from build123d import *

# Parameters (mm, degrees)
CIRCLE001_R            = 0.99
EXTRUDE060_DEPTH       = 4
CIRCLE002_R            = 0.98
EXTRUDE059_DEPTH       = 4
CIRCLE003_R            = 0.99
EXTRUDE058_DEPTH       = 4
CIRCLE004_R            = 0.98
EXTRUDE057_DEPTH       = 4
CIRCLE051_R            = 3.5
EXTRUDE056_DEPTH       = 1.5
EXTRUDE055_DEPTH       = 2.5
CIRCLE049_R            = 2.6
EXTRUDE052_DEPTH       = 1.5
CIRCLE048_R            = 2.6
EXTRUDE051_DEPTH       = 1.5
CIRCLE047_R            = 2.6
EXTRUDE050_DEPTH       = 1.5
CIRCLE050_R            = 2.6
EXTRUDE049_DEPTH       = 1.5
CIRCLE045_R            = 1.5
EXTRUDE045_DEPTH       = 4
CIRCLE043_R            = 1.5
EXTRUDE046_DEPTH       = 4
CIRCLE046_R            = 1.5
EXTRUDE047_DEPTH       = 4
CIRCLE044_R            = 1.5
EXTRUDE048_DEPTH       = 4
CIRCLE040_R            = 23.5
EXTRUDE044_DEPTH       = 4
CUT015_PLACEMENT_ANGLE = 45
CUT018_PLACEMENT_ANGLE = 180


with BuildPart() as extrude060:
    # Circle001 → Extrude060 (new body)
    with BuildSketch(Plane(origin=(100.138196, 1.761986, -7), x_dir=(1, 0, 0), z_dir=(0, 0, -1))):
        Circle(CIRCLE001_R)
    extrude(amount=-EXTRUDE060_DEPTH)


with BuildPart() as extrude059:
    # Circle002 (on Circle) → Extrude059 (new body)
    with BuildSketch(Plane(origin=(104.140973, 1.752854, -7), x_dir=(1, 0, 0), z_dir=(0, 0, -1))):
        Circle(CIRCLE002_R)
    extrude(amount=-EXTRUDE059_DEPTH)


with BuildPart() as extrude058:
    # Circle003 (on Circle) → Extrude058 (new body)
    with BuildSketch(Plane(origin=(121.638501, 1.757256, -7), x_dir=(1, 0, 0), z_dir=(0, 0, -1))):
        Circle(CIRCLE003_R)
    extrude(amount=-EXTRUDE058_DEPTH)


with BuildPart() as extrude057:
    # Circle004 → Extrude057 (new body)
    with BuildSketch(Plane(origin=(125.641919, 1.759529, -7), x_dir=(1, 0, 0), z_dir=(0, 0, -1))):
        Circle(CIRCLE004_R)
    extrude(amount=-EXTRUDE057_DEPTH)


with BuildPart() as extrude056:
    # Circle051 → Extrude056 (new body)
    with BuildSketch(Plane(origin=(115.082764, -1.512482, 32.5), x_dir=(1, 0, 0), z_dir=(0, 0, 1))):
        Circle(CIRCLE051_R)
    extrude(amount=EXTRUDE056_DEPTH)


with BuildPart() as fusion016:
    # Wire001 → Extrude055 (new body)
    with BuildSketch(Plane(origin=(418.588715, 55.5117, 32.5), x_dir=(1, 0, 0), z_dir=(0, 0, 1))):
        Polygon((0, 0), (-11.754715, 1.0599), (-12.322327, 1.134499), (-12.902222, 1.374699), (-13.400116, 1.756802), (-14.0224, 2.834702), (-14.104401, 3.456902), (-14.0224, 4.079201), (-13.782227, 4.6591), (-13.400116, 5.157001), (-12.902283, 5.539154), (-12.322998, 5.780178), (-11.755127, 5.854), (0, 6.913898), (0, 9.889698), (0.077576, 10.479198), (0.31778, 11.059101), (0.69989, 11.557003), (1.197784, 11.939098), (1.777679, 12.179302), (2.399994, 12.261303), (3.022186, 12.179302), (3.602081, 11.939098), (4.100098, 11.557003), (4.482178, 11.059101), (4.722382, 10.479198), (4.799988, 9.889698), (4.799988, 7.405499), (19.059692, 5.853401), (19.622192, 5.779301), (20.202087, 5.539101), (20.601379, 5.2327), (21.082184, 4.6591), (21.322388, 4.079201), (21.404297, 3.456902), (21.322388, 2.834702), (21.082184, 2.254799), (20.601379, 1.681099), (20.202087, 1.374699), (19.622192, 1.134499), (19.059692, 1.060501), (4.799988, -0.4916), (4.799988, -2.9758), (4.722382, -3.5653), (4.482178, -4.145199), (4.100098, -4.6432), (3.602081, -5.025299), (3.022186, -5.265499), (2.398834, -5.366161), (1.777679, -5.265499), (1.197784, -5.025299), (0.69989, -4.6432), (0.31778, -4.145199), (0.077576, -3.5653), (0, -2.9758), align=None)
    extrude(amount=EXTRUDE055_DEPTH)


with BuildPart() as fusion016_1:
    # Extrude055 placement: moved
    add(fusion016.part.moved(Location((-305.905368, -60.481077, -2.5))))

    # Fusion015: union Extrude056
    add(extrude056.part)


with BuildPart() as fusion016_2:
    # Fusion015 placement: moved
    add(fusion016_1.part.moved(Location((-2.193024, 3.267531, -37))))

    # Fusion016: union Extrude060, Extrude059, Extrude058, Extrude057
    add(extrude060.part)
    add(extrude059.part)
    add(extrude058.part)
    add(extrude057.part)


with BuildPart() as fusion016_3:
    # Fusion016 placement: moved
    add(fusion016_2.part.moved(Location((-42.889772, -1.655092, 0))))


with BuildPart() as extrude052:
    # Circle049 → Extrude052 (new body)
    with BuildSketch(Plane(origin=(70, -19.29598, -3), x_dir=(1, 0, 0), z_dir=(0, 0, 1))):
        Circle(CIRCLE049_R)
    extrude(amount=-EXTRUDE052_DEPTH)


with BuildPart() as extrude051:
    # Circle048 → Extrude051 (new body)
    with BuildSketch(Plane(origin=(89.397382, 0.101403, -3), x_dir=(1, 0, 0), z_dir=(0, 0, 1))):
        Circle(CIRCLE048_R)
    extrude(amount=-EXTRUDE051_DEPTH)


with BuildPart() as extrude050:
    # Circle047 (on Cut) → Extrude050 (new body)
    with BuildSketch(Plane(origin=(70, 19.498785, -3), x_dir=(1, 0, 0), z_dir=(0, 0, 1))):
        Circle(CIRCLE047_R)
    extrude(amount=-EXTRUDE050_DEPTH)


with BuildPart() as extrude049:
    # Circle050 → Extrude049 (new body)
    with BuildSketch(Plane(origin=(50.602618, 0.101403, -3), x_dir=(1, 0, 0), z_dir=(0, 0, 1))):
        Circle(CIRCLE050_R)
    extrude(amount=-EXTRUDE049_DEPTH)


with BuildPart() as extrude045:
    # Circle045 → Extrude045 (new body)
    with BuildSketch(Plane(origin=(50.602618, 0.101403, -3), x_dir=(1, 0, 0), z_dir=(0, 0, 1))):
        Circle(CIRCLE045_R)
    extrude(amount=-EXTRUDE045_DEPTH)


with BuildPart() as extrude046:
    # Circle043 → Extrude046 (new body)
    with BuildSketch(Plane(origin=(70, 19.498785, -3), x_dir=(1, 0, 0), z_dir=(0, 0, 1))):
        Circle(CIRCLE043_R)
    extrude(amount=-EXTRUDE046_DEPTH)


with BuildPart() as extrude047:
    # Circle046 → Extrude047 (new body)
    with BuildSketch(Plane(origin=(89.397382, 0.101403, -3), x_dir=(1, 0, 0), z_dir=(0, 0, 1))):
        Circle(CIRCLE046_R)
    extrude(amount=-EXTRUDE047_DEPTH)


with BuildPart() as extrude048:
    # Circle044 → Extrude048 (new body)
    with BuildSketch(Plane(origin=(70, -19.29598, -3), x_dir=(1, 0, 0), z_dir=(0, 0, 1))):
        Circle(CIRCLE044_R)
    extrude(amount=-EXTRUDE048_DEPTH)


with BuildPart() as cut0_disk:
    # Circle040 (on Fusion) → Extrude044 (new body)
    with BuildSketch(Plane(origin=(70, 0.1, -3), x_dir=(1, 0, 0), z_dir=(0, 0, -1))):
        Circle(CIRCLE040_R)
    extrude(amount=EXTRUDE044_DEPTH)

    # Cut008: cut Extrude048
    add(extrude048.part, mode=Mode.SUBTRACT)

    # Cut009: cut Extrude047
    add(extrude047.part, mode=Mode.SUBTRACT)

    # Cut010: cut Extrude046
    add(extrude046.part, mode=Mode.SUBTRACT)

    # Cut011: cut Extrude045
    add(extrude045.part, mode=Mode.SUBTRACT)

    # Cut012: cut Extrude049
    add(extrude049.part, mode=Mode.SUBTRACT)

    # Cut013: cut Extrude050
    add(extrude050.part, mode=Mode.SUBTRACT)

    # Cut014: cut Extrude051
    add(extrude051.part, mode=Mode.SUBTRACT)

    # Cut015: cut Extrude052
    add(extrude052.part, mode=Mode.SUBTRACT)


with BuildPart() as cut0_disk_1:
    # Cut015 placement: moved
    add(cut0_disk.part.moved(Location((20.573185, -49.468206, 0))).rotate(Axis((20.573185, -49.468206, 0), (0, 0, 1)), CUT015_PLACEMENT_ANGLE))

    # Cut018: cut Fusion016
    add(fusion016_3.part, mode=Mode.SUBTRACT)


with BuildPart() as cut0_disk_2:
    # Cut018 placement: moved
    add(cut0_disk_1.part.moved(Location((-27.831247, -11.66637, 3.7))).rotate(Axis((-27.831247, -11.66637, 3.7), (1, 0, 0)), CUT018_PLACEMENT_ANGLE))


solid = cut0_disk_2.part
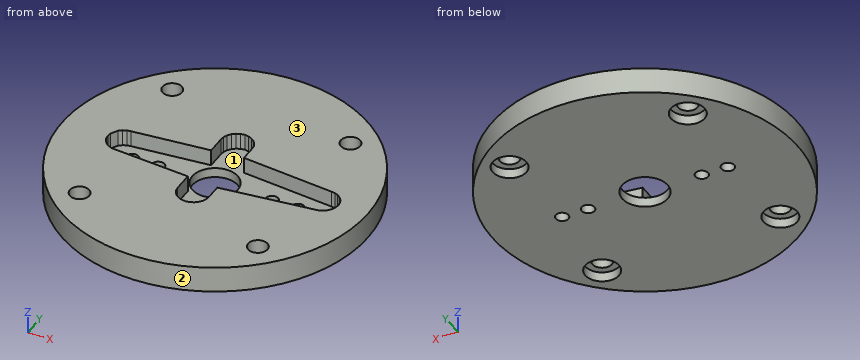
Input: part model. Units: mm. Frame: model coordinates. Face numbers are marked on the shaded views. Coordinates: 2 decimals unless noted, no trailing zeros. Loops run counter-clockwise (first coordinate to the right, second up) from the corner with the lowest first, then second, coordinate; pieces in that order, holes last. Notation, with made-up numbers: (38.5, 69) -> (70.5, 69) arc R23 cw to (70.5, 93) -> close; hole circle Ø6 at (55, 86.25). An arc over 180 degrees is marked (long way). Write item = value, one per line. Start each with the question number.
Item 1: Cut plane B-B, the plane z = 7.5. Count the separate pieces of the cut face and the enclosed holes in it, plus the area to 3 significant figures.
Item 2: Cut plane A-A, the plane y = -26. Return loops of the section in (x, z), plus the area to 3 significant figures.
Item 3: First-contact query: P1, Ø2.5, axis at x = 28.5, y = 1, coming from the -Z side; P2, Ø2, axis at y = -16.5, z = 8, coming from the -X side; P3, Ø1, axis at x = 49, y = -11, coming from the +Z side. Flat tips, straight axial feed; report the tip coordinate or a pass-through.
Item 4: Cut plane C-C, the plane x = 48.5. Return loops of the section in (y, z), plus the area to 3 significant figures.
Item 5: Mould query, pull axis X, two halves, no side actions, for the marked faces 1, 2 and 3. Classes: pulls with the +X half, pulls with the -X half, needs draft (parallel to the pull), parting line crosses it, or undercut.
Item 6: Material intervals for line 1 (X direction, y = 2.5, z = 10.1); line 2 (X direction, y = 4, z = 8.1); line 3 (Y direction, x = 37, z = 8.3), sorted ascending.
Ans:
q1.separate_pieces = 1
q1.enclosed_holes = 9
q1.area = 1,600 mm²
q2.outline = (23.47, 6.7) -> (25.9, 6.7) -> (25.9, 8.2) -> (27.04, 8.2) -> (27.04, 10.7) -> (23.47, 10.7) -> close; (29.86, 8.2) -> (31, 8.2) -> (31, 6.7) -> (53.34, 6.7) -> (53.34, 8.2) -> (54.48, 8.2) -> (54.48, 10.7) -> (29.86, 10.7) -> close; (57.29, 8.2) -> (58.43, 8.2) -> (58.43, 6.7) -> (60.87, 6.7) -> (60.87, 10.7) -> (57.29, 10.7) -> close
q2.area = 120 mm²
q3.P1 = 8.2
q3.P2 = 18.97
q3.P3 = 8.2
q4.outline = (-34.4, 6.7) -> (10.86, 6.7) -> (10.86, 10.7) -> (-8.25, 10.7) -> (-8.25, 8.2) -> (-15.29, 8.2) -> (-15.29, 10.7) -> (-34.4, 10.7) -> close
q4.area = 163 mm²
q5.face_1 = undercut
q5.face_2 = parting line crosses it
q5.face_3 = needs draft
q6.line_1 = 23.49 to 27.06, 29.85 to 54.49, 57.28 to 60.84
q6.line_2 = 24.74 to 26.85, 30.05 to 54.29, 57.48 to 59.59
q6.line_3 = -34.69 to -14.97, -8.56 to 11.16
